Could you check a few things on this drawing? It's one solid part, dimensions in mm from its lowest x, y, z. Give positions to 0.01 mm unless a question says otherwise; leave off trailing zeros. Order: outer loops, then holes, each group sorted by start corner. A loop starts at its lowest first (then second) coordinate and runs counter-clockwise, first axis right, second up. Notation, with made-up numbers: (34, 77) - (92, 77) arc R18 cw to (92, 109) - close; hole circle Ø11 at (74, 71). An arc over 180 degrees is marked (long way). Return JSON: item names as keys, results as strings.
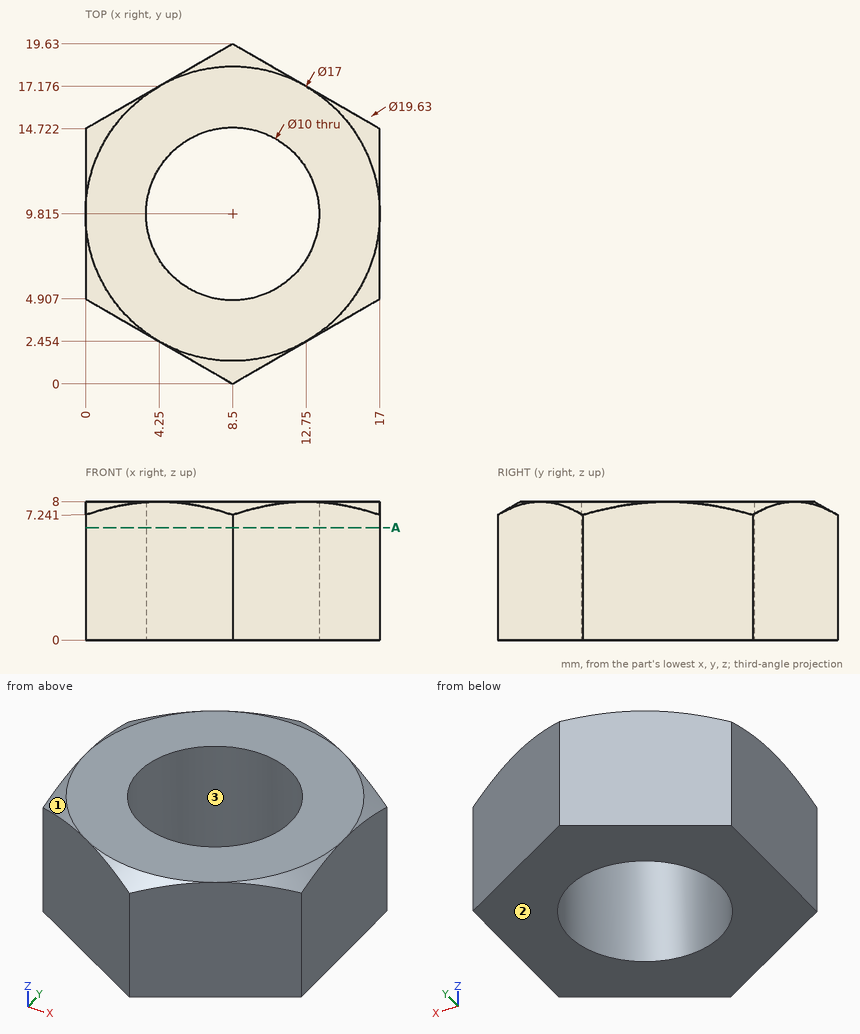
1. Thinking about a two-plate mould opening in X: for the marked faces 1, 2 and 3, which applies, +X half, -X half, draft (parallel to the pull), parting line (faces both ways), or undercut?
Checks:
{"face 1": "-X half", "face 2": "draft", "face 3": "undercut"}
2. Suppose I cut it at A-A (z = 6.5). List the corners of the cut face in (x, y) for me (1 decimal).
Checks:
{"outline": "(0, 4.9) - (8.5, 0) - (17, 4.9) - (17, 14.7) - (8.5, 19.6) - (0, 14.7) - close; hole circle Ø10 at (8.5, 9.8)"}
3. For pin 1 Ø1 at (y, z) = (3.5, 3) entering from +X, with a flat end and sliding along its axis, tell me the tip position at first contact or that it passes through.
Checks:
{"pin 1": "x = 15.43"}
4. If I drill on L1, parallel to Y at x = 7.75, z = 1.75 (1 decimal); L2, parallel to Y at x = 11.75, z = 7.25 (1 decimal); L3, parallel to X at y = 9.5, z = 0.75, over which ranges is the centre line in solid material (lowest first)? Write a range as [from, to].
Checks:
{"L1": "[0.4, 4.9], [14.8, 19.2]", "L2": "[1.9, 6], [13.6, 17.8]", "L3": "[0, 3.51], [13.49, 17]"}
